The listing builds one solid part. Answer for the finished solid, in the listing's coordinates (mm). Give positions to 0.01 mm unless a question says otherwise; leave off trailing zeros. Write each loop counter-clockwise with the first axis right and the second up, starting at its lowest first coordinate (ties: lowest second). Pieces come first, ordered by that corner, then holes. Notation, with made-up numbers: (-5.5, 7.25) - (6.5, 7.25) arc R15 ccw to (6.5, 23.25) - close; hole circle Ø4 at (-40, 35). An arc over 180 degrees is marked (long way). Answer as CSV lines item,"result". Start each with the question number.
(1) Find section C-C (x = 99). Write down the section's boundary in (y, z).
(2) Each of these flat-tipped pins is pushed along its axis until it touches: pin 1 Ø0.8 at (y, z) = (-1, 0.5) entering from -X; pin 2 Ø5 at (x, y) = (119.5, -2) entering from -Z; pin 3 Ø0.8 at (y, z) = (-1, 1) entering from +X. Where does it stop, or does it pass through?
(3) Find section B-B (y = -1). Write down the section's boundary in (x, z), then the cut area to 3 significant figures.
(4) Find section D-D (y = -9.25). Write down the section's boundary in (x, z).
(5) Straight lines are drawn through the part: probe 1 along X at (y, z) = (-4.75, 1.2); probe 2 along X at (y, z) = (-6, 1.25); probe 3 along X at (y, z) = (-0.25, 0.25). For each, find the intervals that lie inside material, in ascending order.
(6) Find section A-A (x = 106.5). Write down the section's boundary in (y, z).
from build123d import *

# Parameters (mm, degrees)
BOSS_EXTRUDE1_DEPTH = 1.524


with BuildPart() as part:
    # Sketch1 → Boss-Extrude1 (new body)
    with BuildSketch(Plane.XY):
        with BuildLine():
            Line((106.811293612, -4.205619723), (105.503930304, -1.524))
            Line((105.503930304, -1.524), (106.800157748, -1.524))
            Line((106.800157748, -1.524), (106.800157748, 0))
            Line((106.800157748, 0), (108.32415775, 0))
            Line((108.32415775, 0), (108.32415775, -1.524))
            Line((108.32415775, -1.524), (109.620385194, -1.524))
            Line((109.620385194, -1.524), (108.313021885, -4.205619723))
            ThreePointArc((108.313021885, -4.205619723), (108.616799976, -5.654511508), (109.13336302, -7.041858312))
            ThreePointArc((109.13336302, -7.041858312), (111.286278886, -8.804119786), (114.000740009, -8.193945187))
            ThreePointArc((114.000740009, -8.193945187), (117.860186741, -2.977615774), (118.628372854, 3.4656219))
            Line((118.628372854, 3.4656219), (120.110575877, 4.061475664))
            Line((120.110575877, 4.061475664), (119.542132666, 5.475494164))
            Line((119.542132666, 5.475494164), (120.956151165, 6.043937374))
            Line((120.956151165, 6.043937374), (121.524594376, 4.629918875))
            Line((121.524594376, 4.629918875), (123.006797398, 5.225772639))
            ThreePointArc((123.006797398, 5.225772639), (122.943528087, 2.333705851), (122.428113191, -0.512765789))
            Line((122.428113191, -0.512765789), (121.057887131, 0.088329507))
            Line((121.057887131, 0.088329507), (120.639136812, -1.392165095))
            Line((120.639136812, -1.392165095), (121.97564456, -1.97846873))
            ThreePointArc((121.97564456, -1.97846873), (119.201094938, -7.067703715), (114.981972786, -11.042303895))
            Line((114.981972786, -11.042303895), (114.195536637, -9.777044843))
            Line((114.195536637, -9.777044843), (112.901190835, -10.581560192))
            Line((112.901190835, -10.581560192), (113.687626985, -11.846819244))
            ThreePointArc((113.687626985, -11.846819244), (110.720377701, -13.193789782), (107.562157749, -13.996625182))
            ThreePointArc((107.562157749, -13.996625182), (104.403937797, -13.193789782), (101.436688513, -11.846819244))
            Line((101.436688513, -11.846819244), (102.223124662, -10.581560192))
            Line((102.223124662, -10.581560192), (100.928778861, -9.777044843))
            Line((100.928778861, -9.777044843), (100.142342712, -11.042303895))
            ThreePointArc((100.142342712, -11.042303895), (95.923220559, -7.067703715), (93.148670938, -1.97846873))
            Line((93.148670938, -1.97846873), (94.485178686, -1.392165095))
            Line((94.485178686, -1.392165095), (94.066428367, 0.088329507))
            Line((94.066428367, 0.088329507), (92.696202307, -0.512765789))
            ThreePointArc((92.696202307, -0.512765789), (92.18078741, 2.333705851), (92.117518099, 5.225772639))
            Line((92.117518099, 5.225772639), (93.599721122, 4.629918875))
            Line((93.599721122, 4.629918875), (94.168164333, 6.043937374))
            Line((94.168164333, 6.043937374), (95.582182832, 5.475494164))
            Line((95.582182832, 5.475494164), (95.013739621, 4.061475664))
            Line((95.013739621, 4.061475664), (96.495942644, 3.4656219))
            ThreePointArc((96.495942644, 3.4656219), (97.264128757, -2.977615774), (101.123575488, -8.193945187))
            ThreePointArc((101.123575488, -8.193945187), (103.838036611, -8.804119786), (105.990952478, -7.041858312))
            ThreePointArc((105.990952478, -7.041858312), (106.507515522, -5.654511508), (106.811293612, -4.205619723))
        make_face()
    extrude(amount=BOSS_EXTRUDE1_DEPTH)


solid = part.part
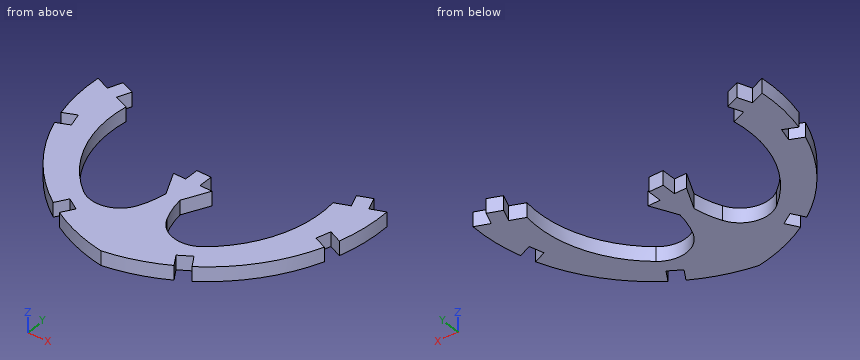
Result set:
1,outline,"(-10.2, 0) - (-6.03, 0) - (-6.03, 1.52) - (-10.2, 1.52) - close"
2,pin 1,"x = 94.26"
2,pin 2,"z = 0"
2,pin 3,"x = 120.86"
3,outline,"(94.37, 0) - (96.66, 0) - (96.66, 1.52) - (94.37, 1.52) - close; (106.8, 0) - (108.32, 0) - (108.32, 1.52) - (106.8, 1.52) - close; (118.46, 0) - (120.75, 0) - (120.75, 1.52) - (118.46, 1.52) - close"
3,area,"9.29 mm^2"
4,outline,"(97.91, 0) - (117.22, 0) - (117.22, 1.52) - (97.91, 1.52) - close"
5,probe 1,"94.4 to 98.13, 106.72 to 108.4, 116.99 to 120.73"
5,probe 2,"95.16 to 98.98, 106.4 to 108.72, 116.15 to 119.97"
5,probe 3,"92.63 to 93.3, 94.16 to 96.52, 106.8 to 108.32, 118.6 to 120.96, 121.83 to 122.5"
6,outline,"(-13.79, 0) - (-5.68, 0) - (-5.68, 1.52) - (-13.79, 1.52) - close; (-3.57, 0) - (-1.52, 0) - (-1.52, 1.52) - (-3.57, 1.52) - close"
